from build123d import *

# Parameters (mm, degrees)
SKETCH1_W               = 40
SKETCH1_H               = 2
CUT_EXTRUDE1_DEPTH      = 41.099875312
CUT_EXTRUDE1_DEPTH_BACK = 41.099875312
CUT_EXTRUDE2_START      = 1.5
SKETCH3_W               = 4
SKETCH3_H               = 5.7
CUT_EXTRUDE2_DEPTH      = 39.599875421
SKETCH4_W               = 2.5
SKETCH4_H               = 3.175
CUT_EXTRUDE3_DEPTH      = 41.099875421


with BuildPart() as part:
    # Sketch1 → Revolve1 (revolve)
    with BuildSketch(Plane(origin=(0, 0, 0), x_dir=(0, 0, -1), z_dir=(1, 0, 0)), mode=Mode.PRIVATE) as revolve1_sk:
        with Locations((-20, 1)):
            Rectangle(SKETCH1_W, SKETCH1_H)
    revolve(revolve1_sk.sketch.rotate(Axis((0, 0, -0.721189591), (0, 0, -1)), 90), axis=Axis((0, 0, -0.721189591), (0, 0, -1)))

    # Sketch2 → Cut-Extrude1 (cut, two sides: drawn at the far end of the back side and taken through both)
    with BuildSketch(Plane(origin=(0, 0, 0), x_dir=(1, 0, 0), z_dir=(0, 1, 0)).offset(-CUT_EXTRUDE1_DEPTH_BACK)):
        with BuildLine():
            Line((-1.25, 0), (-1.25, -5))
            ThreePointArc((-1.25, -5), (-2.17993597, -7.24506403), (-4.425, -8.175))
            Line((-4.425, -8.175), (-4.425, 0))
            Line((-4.425, 0), (-1.25, 0))
        make_face()
        with BuildLine():
            Line((1.25, 0), (1.25, -5))
            ThreePointArc((1.25, -5), (2.17993597, -7.24506403), (4.425, -8.175))
            Line((4.425, -8.175), (4.425, 0))
            Line((4.425, 0), (1.25, 0))
        make_face()
    extrude(amount=CUT_EXTRUDE1_DEPTH + CUT_EXTRUDE1_DEPTH_BACK, mode=Mode.SUBTRACT)

    # Sketch3 → Cut-Extrude2 (cut, through all)
    with BuildSketch(Plane(origin=(0, 0, 0), x_dir=(1, 0, 0), z_dir=(0, 1, 0)).offset(CUT_EXTRUDE2_START)):
        with Locations((0, -2.85)):
            Rectangle(SKETCH3_W, SKETCH3_H)
    extrude(amount=CUT_EXTRUDE2_DEPTH, mode=Mode.SUBTRACT)

    # Sketch4 → Cut-Extrude3 (cut, through all)
    with BuildSketch(Plane(origin=(0, 0, 0), x_dir=(1, 0, 0), z_dir=(0, 1, 0))):
        with Locations((0, -3.0875)):
            Rectangle(SKETCH4_W, SKETCH4_H)
    extrude(amount=CUT_EXTRUDE3_DEPTH, mode=Mode.SUBTRACT)


solid = part.part
CAD build for the part. Positions are in the model's coordinates, mm. A direction names the side the tool comes from. Coordinates: 2 decimals unless noted, no trailing zeros. Write each loop counter-clockwise with the first axis right and the second up, starting at its lowest first coordinate (ties: lowest second). Pieces come first, ordered by that corner, then holes. Notation, with made-up numbers: M 80,-25.75 L 102,-25.75 A25 cw 102,8.25 Z; hole C 44.5,31.5 d8. An arc over 180 degrees is marked long. Answer as a JSON object with one key per item and string values. Group by question number.
1) Saw through at D-D (y = -0.9). Write the cut outline in (x, z) (3 decimals), plus the area to 3 significant figures.
2) Saw through at A-A (y = 0.95). Write the cut outline in (x, z) (3 decimals).
3) Pin check, flat tips, straight feed: pin 1 Ø2 at (x, z) = (1.5, 5) entering from -Y; pin 2 Ø0.8 at (x, z) = (-0.5, 2.5) entering from +Y; pin 3 Ø1.1 at (x, z) = (-0.5, 5) entering from +Y. Stop position of each tip, or through.
4) Saw through at B-B (x = 0). Write the cut outline in (y, z) (3 decimals).
5) Wall check: line 1 (Z direction, x = -0.25, y = 0.65) (3 decimals); line 2 (Y direction, x = -0.15, z = 3.5); line 3 (X direction, y = 1.15, z = 5). Give the ranges that are in metal, low to high. Write a range as from..to.
6) Mould opens along Z. For faces 1 (the face through (-1.363, -0.052, 5.841)), 2 (the face through (0, -2, 24)), 3 (the face through (0, 1, 4.675)) say: +Z half, -Z half, draft (parallel to the pull), parting line (faces both ways), or undercut.
7) Saw through at C-C (z = 33.5). Write the cut outline in (x, y).
8) Tool access for faces 4 (the face through (1.25, -0.4, 2.5)), 5 (the face through (0, 1.5, 5)), 6 (the face through (0, 0, 3)): list every direction of +Z, -Z, +X, -X, +Y, -Y with a clear straight run to the whole face (end or side of a thin tool).
Values follow:
{
 "1": {"outline": "M -1.786,6.765 A3.175 cw -1.25,5 L -1.25,0 L 1.25,0 L 1.25,5 A3.175 cw 1.786,6.765 L 1.786,40 L -1.786,40 Z", "area": "136 mm2"},
 "2": {"outline": "M -1.76,6.726 A3.175 cw -1.25,5 L -1.25,4.675 L 1.25,4.675 L 1.25,5 A3.175 cw 1.76,6.726 L 1.76,40 L -1.76,40 Z; M -1.25,0 L 1.25,0 L 1.25,1.5 L -1.25,1.5 Z"},
 "3": {"pin 1": "stops at y = -1.94", "pin 2": "stops at y = 0", "pin 3": "stops at y = 1.5"},
 "4": {"outline": "M -2,0 L 1.5,0 L 1.5,1.5 L 0,1.5 L 0,4.675 L 1.5,4.675 L 1.5,5.7 L 2,5.7 L 2,40 L -2,40 Z"},
 "5": {"line 1": "z = 0..1.5, 4.675..40", "line 2": "y = -1.99..0", "line 3": "x = -1.25..1.25"},
 "6": {"face 1": "-Z half", "face 2": "draft", "face 3": "undercut"},
 "7": {"outline": "C 0,0 d4"},
 "8": {"face 4": "-Z, +X, +Y, -Y", "face 5": "-Z, +X, -X, +Y", "face 6": "+X, -X, +Y"}
}
